Source: CAD feature listing. Evaluate the final solid. Frame: model axes, mm. A direction names the side the tool comes from. Coordinates: 2 decimals unless noted, no trailing zeros. Order: outer loops, then holes, each group sorted by start corner. A loop starts at its lowest first (then second) coordinate and runs counter-clockwise, first axis right, second up. Notation, with made-up numbers: (84.5, 60.5) -> (134.5, 60.5) arc R11 cw to (134.5, 77.5) -> close; hole circle Ø1 at (33, 65). An arc over 180 degrees is marked (long way). Put each result on its own line as item: value.
from build123d import *

# Parameters (mm, degrees)
F0_W      = 65
F0_H      = 65
F1_DEPTH  = 15
F2_R      = 18.25
F3_DEPTH  = 4.2
F4_R      = 10
F5_DEPTH  = 25
F6_R      = 5
F7_DEPTH  = 10
F8_R      = 2
F9_DEPTH  = 25
F12_R     = 5
F13_DEPTH = 11
F11_R     = 2
F14_DEPTH = 25
F15_R     = 2
F16_DEPTH = 7


with BuildPart() as f1:
    # F0 (on Front) → F1 (new body)
    with BuildSketch(Plane.XZ):
        Rectangle(F0_W, F0_H)
    extrude(amount=F1_DEPTH)

    # F2 (on face) → F3 (cut)
    with BuildSketch(Plane.XZ.offset(15)):
        Circle(F2_R)
    extrude(amount=-F3_DEPTH, mode=Mode.SUBTRACT)

    # F4 (on face) → F5 (cut)
    with BuildSketch(Plane.XZ.offset(15)):
        Circle(F4_R)
    extrude(amount=-F5_DEPTH, mode=Mode.SUBTRACT)

    # F6 (on face) → F7 (cut)
    with BuildSketch(Plane.XZ.offset(15)):
        with BuildLine():
            ThreePointArc((15, -22.5), (10, -17.5), (5, -22.5))
            ThreePointArc((5, -22.5), (10, -27.5), (15, -22.5))
        make_face()
        with Locations((-10, -22.5)):
            Circle(F6_R)
    extrude(amount=-F7_DEPTH, mode=Mode.SUBTRACT)

    # F8 (on face) → F9 (cut)
    with BuildSketch(Plane.XZ.offset(15)):
        with Locations((-10, -22.5)):
            Circle(F8_R)
        with Locations((10, -22.5)):
            Circle(F8_R)
    extrude(amount=-F9_DEPTH, mode=Mode.SUBTRACT)

    # F12 (on face) → F13 (cut)
    with BuildSketch(Plane(origin=(0, 0, 0), x_dir=(-1, 0, 0), z_dir=(0, 1, 0))):
        with Locations((18.616408, 18.859463)):
            Circle(F12_R)
        with Locations((18.995447, -18.477634)):
            Circle(F12_R)
        with Locations((-18.859462, -18.616409)):
            Circle(F12_R)
        with Locations((-18.75598, 18.720663)):
            Circle(F12_R)
    extrude(amount=-F13_DEPTH, mode=Mode.SUBTRACT)

    # F11 (on face) → F14 (cut)
    with BuildSketch(Plane.XZ.offset(15)):
        with Locations((-18.73833, 18.73833)):
            Circle(F11_R)
        with Locations((-18.73833, -18.73833)):
            Circle(F11_R)
        with Locations((18.73833, 18.73833)):
            Circle(F11_R)
        with Locations((18.73833, -18.73833)):
            Circle(F11_R)
    extrude(amount=-F14_DEPTH, mode=Mode.SUBTRACT)

    # F15 (on face) → F16 (cut)
    with BuildSketch(Plane(origin=(0, 0, -32.5), x_dir=(1, 0, 0), z_dir=(0, 0, -1))):
        with BuildLine():
            ThreePointArc((8, 2.5), (8.585786, 1.085786), (10, 0.5))
            Line((10, 0.5), (10, 2.5))
            Line((10, 2.5), (8, 2.5))
        make_face()
        with Locations((-10, 2.5)):
            Circle(F15_R)
        with BuildLine():
            Line((10, 2.5), (10, 0.5))
            ThreePointArc((10, 0.5), (11.414214, 1.085786), (12, 2.5))
            ThreePointArc((12, 2.5), (10, 4.5), (8, 2.5))
            Line((8, 2.5), (10, 2.5))
        make_face()
    extrude(amount=-F16_DEPTH, mode=Mode.SUBTRACT)


solid = f1.part
1. First-contact query: pin 1 (8 mm diameter, centred on x = 18.76, z = 18.72, fed in from +Y); pin 2 (18 mm diameter, centred on x = 8, z = -2, fed in from -Y). Flat tips, straight axial feed; report the tip coordinate or a pass-through.
Numbers:
pin 1: stops at y = -11
pin 2: stops at y = -10.8
2. Cut plane D-D on y = -9. Output: boundary loops of the cut face in (x, z), plus the area to 3 significant figures.
Numbers:
outline: (-32.5, -32.5) -> (32.5, -32.5) -> (32.5, 32.5) -> (-32.5, 32.5) -> close; hole circle Ø10 at (-18.62, 18.86); hole (-14.85, -21.27) arc R5 ccw (long way) to (-14.15, -19.71) arc R5 ccw (long way) to start; hole circle Ø20 at (0, 0); hole circle Ø10 at (18.76, 18.72); hole (13.92, -19.4) arc R5 ccw (long way) to (14.94, -21.72) arc R5 ccw (long way) to start
area: 3,440 mm2
3. Cut plane A-A on x = 0. Output: boundary loops of the cut face in (y, z).
Numbers:
outline: (-15, -32.5) -> (0, -32.5) -> (0, -10) -> (-10.8, -10) -> (-10.8, -18.25) -> (-15, -18.25) -> close; (-15, 18.25) -> (-10.8, 18.25) -> (-10.8, 10) -> (0, 10) -> (0, 32.5) -> (-15, 32.5) -> close
4. Cut plane C-C on x = -17.5. Output: boundary loops of the cut face in (y, z), plus the area to 3 significant figures.
Numbers:
outline: (-15, -32.5) -> (0, -32.5) -> (0, -23.25) -> (-11, -23.25) -> (-11, -20.31) -> (-15, -20.31) -> close; (-15, -17.17) -> (-11, -17.17) -> (-11, -13.71) -> (0, -13.71) -> (0, 13.99) -> (-11, 13.99) -> (-11, 17.17) -> (-15, 17.17) -> (-15, 5.18) -> (-10.8, 5.18) -> (-10.8, -5.18) -> (-15, -5.18) -> close; (-15, 20.31) -> (-11, 20.31) -> (-11, 23.73) -> (0, 23.73) -> (0, 32.5) -> (-15, 32.5) -> close
area: 694 mm2
5. Pull-direction query (X, two-part tool) for faces 1 (the cylindrical face through (-7.693, -10.07, -26.936)), 2 (the flat face through (-32.5, -7, 0)), 3 (the flat face through (-8, 0, -7)), 4 (the flat face through (19, -11, -21)); classes: pulls with the +X half, pulls with the -X half, needs draft (parallel to the pull), parting line crosses it, or undercut.
Numbers:
face 1: undercut
face 2: pulls with the -X half
face 3: needs draft
face 4: undercut
6. Cut plane B-B on z = 0. Output: boundary loops of the cut face in (x, y).
Numbers:
outline: (-32.5, -15) -> (-18.25, -15) -> (-18.25, -10.8) -> (-10, -10.8) -> (-10, 0) -> (-32.5, 0) -> close; (10, -10.8) -> (18.25, -10.8) -> (18.25, -15) -> (32.5, -15) -> (32.5, 0) -> (10, 0) -> close
7. Set-up query: faces 5 (the flat face through (10, -3, -25.5)), 6 (the cylindrical face through (5.23, -10.07, -24)), 7 (the flat face through (0, -7, 32.5)), 8 (the cylindrical face through (-18.34, -5.42, -13.52)). Return all of +Z, -Z, +X, -X, +Y, -Y with unobstructed straight access to the full face (end or side cutting, diameter ignored); none if empty.
Numbers:
face 5: -Z
face 6: -Y
face 7: +Z, +X, -X, +Y, -Y
face 8: +Y
8. Ray query, line 1 along X through (y, z) = (-13.25, 19); line 2 along Z through (x, y) = (9.5, -11.5); line 3 along Z through (x, y) = (23, -5.25). Return the intervals inside material, ascending.
Numbers:
line 1: x = -32.5 to -20.72, -16.76 to 16.76, 20.72 to 32.5
line 2: z = -32.5 to -27.47, -17.53 to -15.58, 15.58 to 32.5
line 3: z = -32.5 to -21.42, -15.81 to 16.08, 21.36 to 32.5
